```python
from build123d import *

# Parameters (mm, degrees)
F3_R = 1.5875


with BuildPart() as f2:
    # F2: sweep along a path in F1
    with BuildLine(Plane.XY) as f2_path:
        Line((0, 0), (0, 44.45))
        ThreePointArc((0, 44.45), (1.8598719395, 48.9401280605), (6.35, 50.8))
        Line((6.35, 50.8), (25.4, 50.8))
    # F0 (on Front) → F2 (sweep)
    with BuildSketch(Plane.XZ):
        Polygon((3.175, -1.8330871047), (3.175, 1.8330871047), (0, 3.6661742094), (-3.175, 1.8330871047), (-3.175, -1.8330871047), (0, -3.6661742094), align=None)
    sweep(path=f2_path.line)

    # F4: sweep along a path in F4_path
    with BuildLine(Plane(origin=(3.175, 0, -1.8330871047), x_dir=(-1, 0, 0), z_dir=(0, 0, 1))) as f4_path:
        Line((0, 0), (0, -44.45))
        ThreePointArc((0, -44.45), (-0.9299359697, -46.6950640303), (-3.175, -47.625))
        Line((-3.175, -47.625), (-22.225, -47.625))
    # F3 (on face) → F4 (sweep, cut)
    with BuildSketch(Plane.XZ):
        Circle(F3_R)
    sweep(path=f4_path.line, mode=Mode.SUBTRACT)


solid = f2.part
```
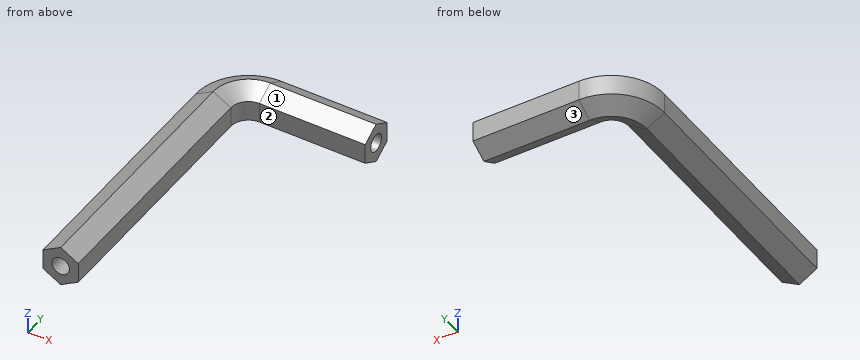
Check sheet for the modelled part. Datum: model origin and axes. Units: mm. Face numbers are marked on the shaded views. A direction names the side the tool comes from. Give positions to 0.01 mm unless a question says otherwise; leave off trailing zeros. Loops run counter-clockwise (first coordinate to the right, second up) from the corner with the lowest first, then second, coordinate; pieces in that order, holes last. Notation, with made-up numbers: M 62,3 L 110,3 A26 ccw 110,23 Z; hole C 56.5,23 d8. An arc over 180 degrees is marked long. Answer as CSV lines item,"result".
Item 1: Sectioned sample at C-C, the plane y = 40. Enter the section's corners in (x, z) (1 decimal).
Reply:
outline,"M -3.2,-1.8 L 0,-3.7 L 3.2,-1.8 L 3.2,1.8 L 0,3.7 L -3.2,1.8 Z; hole C 0,0 d3.2"
Item 2: Scan lines: L1, parallel to Y at x = 10.75, z = 0 (1 decimal); L2, parallel to Z at x = 0, y = 20; L3, parallel to Y at x = 19, z = 0.75 (3 decimals). Record each from-to range of solid material in increasing order.
Reply:
L1,"47.6 to 49.2, 52.4 to 54"
L2,"-3.67 to -1.59, 1.59 to 3.67"
L3,"47.625 to 49.401, 52.199 to 53.975"
Item 3: Sectioned sample at B-B, the plane x = 7.5. Enter the section's corners in (y, z) (1 decimal).
Reply:
outline,"M 47.6,-1.8 L 50.8,-3.7 L 54,-1.8 L 54,1.8 L 50.8,3.7 L 47.6,1.8 Z; hole C 50.8,0 d3.2"
Item 4: Set-up check for the marked faces 1, 2 and 3: record each of +Z, -Z, +X, -X, +Y, -Y from which the full face is reachable in a straight line by a thin tool's end or side.
Reply:
face 1,"+Z, +X, -Y"
face 2,"+Z, -Z, +X, -Y"
face 3,"-Z, +X, -X, +Y"
Item 5: Depth check by flat-ended pin: pin 1 Ø12 at (x, y) = (12.5, 30.5) entering from -Z; pin 2 Ø1 at (x, y) = (1.5, 9) entering from +Z; pin 3 Ø1 at (y, z) = (45.5, 1) entering from +X; pin 4 Ø1.8 at (y, z) = (14, -1) entering from +X (3 decimals). Enter the tip coordinate at first touch or a pass-through.
Reply:
pin 1,"through"
pin 2,"z = 3.09"
pin 3,"x = 3.58"
pin 4,"x = 3.175"
Item 6: Sectioned sample at D-D, the plane z = -2.75. Enter the section's corners in (x, y).
Reply:
outline,"M -1.59,0 L 1.59,0 L 1.59,44.45 A4.76 cw 6.35,49.21 L 25.4,49.21 L 25.4,52.39 L 6.35,52.39 A7.94 ccw -1.59,44.45 Z"
